Source: CAD feature listing. Evaluate the final solid. Frame: model axes, mm. A direction names the side the tool comes from. Give positions to 0.01 mm unless a question says otherwise; leave off trailing zeros. Order: outer loops, then holes, each group sorted by start corner. A loop starts at its lowest first (then second) coordinate and runs counter-clockwise, first axis right, second up.
```python
from build123d import *

# Parameters (mm, degrees)
SKETCH1_W                    = 1080
SKETCH1_H                    = 33
BASE_FLANGE1_DEPTH           = 2
EDGE_FLANGE1_STRIP_W         = 12
EDGE_FLANGE1_STRIP_H         = 2
EDGE_FLANGE1_STRIP_CUT_DEPTH = 1080
EDGE_FLANGE1_DEPTH           = 1080
SKETCH9_R                    = 7
CUT_EXTRUDE1_DEPTH           = 10
CUT_EXTRUDE2_DEPTH           = 40
CUT_EXTRUDE2_DEPTH_BACK      = 40


# Sheet-metal steps are written as plain solids
with BuildPart() as part:
    # Sketch1 → Base-Flange1 (new body)
    with BuildSketch(Plane.XY):
        Rectangle(SKETCH1_W, SKETCH1_H)
    extrude(amount=-BASE_FLANGE1_DEPTH)

    # Edge-Flange1 strip (across the edge) → Edge-Flange1 strip cut (cut)
    with BuildSketch(Plane(origin=(-540, -16.5, 0), x_dir=(0, 1, 0), z_dir=(1, 0, 0))):
        with Locations((-2, -1)):
            Rectangle(EDGE_FLANGE1_STRIP_W, EDGE_FLANGE1_STRIP_H)
    extrude(amount=EDGE_FLANGE1_STRIP_CUT_DEPTH, mode=Mode.SUBTRACT)

    # Edge-Flange1 section (across the edge) → Edge-Flange1 (add)
    with BuildSketch(Plane(origin=(-540, -16.5, 0), x_dir=(0, 1, 0), z_dir=(1, 0, 0))):
        with BuildLine():
            Line((0, 2), (0, 8))
            Line((0, 8), (2, 8))
            Line((2, 8), (2, 2))
            ThreePointArc((2, 2), (2.585786438, 0.585786438), (4, 0))
            Line((4, 0), (4, -2))
            ThreePointArc((4, -2), (1.171572875, -0.828427125), (0, 2))
        make_face()
    extrude(amount=EDGE_FLANGE1_DEPTH)

    # Sketch9 → Cut-Extrude1 (cut)
    with BuildSketch(Plane.XY):
        with Locations((-930, 2)):
            Circle(SKETCH9_R)
        with Locations((-626, 2)):
            Circle(SKETCH9_R)
        with Locations((-322, 2)):
            Circle(SKETCH9_R)
        with Locations((-18, 2)):
            Circle(SKETCH9_R)
        with Locations((286, 2)):
            Circle(SKETCH9_R)
        with Locations((590, 2)):
            Circle(SKETCH9_R)
        with Locations((894, 2)):
            Circle(SKETCH9_R)
    extrude(amount=-CUT_EXTRUDE1_DEPTH, mode=Mode.SUBTRACT)

    # Sketch10 → Cut-Extrude2 (cut, two sides: drawn at the far end of the back side and taken through both)
    with BuildSketch(Plane.XY.offset(-CUT_EXTRUDE2_DEPTH_BACK)):
        Polygon((-302.377446669, -47.622553331), (-401.622553331, 51.622553331), (-590.417878705, 51.622553331), (-583.65364731, -79.056750642), (-558.625991149, -79.056750642), align=None)
        Polygon((558.625991149, -79.056750642), (302.377446669, -47.622553331), (401.622553331, 51.622553331), (590.417878705, 51.622553331), (583.65364731, -79.056750642), align=None)
    extrude(amount=CUT_EXTRUDE2_DEPTH + CUT_EXTRUDE2_DEPTH_BACK, mode=Mode.SUBTRACT)


solid = part.part
```
1) Reachability of faces 1 (the flat face through (-5, 2, 0)), 2 (the flat face through (-5, 2, -2)) from +Z, -Z, +X, -X, +Y, -Y: full face, straight path, thin tool, end or side. Return the list, or none.
Report:
face 1: +Z, +X, -X, +Y
face 2: -Z, +X, -X, +Y, -Y
2) Section query A-A, the plane x = 286. Return the cut outline in (y, z).
Report:
outline: (-16.5, 2) arc R4 ccw to (-12.5, -2) - (-5, -2) - (-5, 0) - (-12.5, 0) arc R2 cw to (-14.5, 2) - (-14.5, 8) - (-16.5, 8) - close; (9, -2) - (16.5, -2) - (16.5, 0) - (9, 0) - close
3) Section query B-B, the plane z = 3.75. Return the cut outline in (x, y).
Report:
outline: (-335.5, -14.5) - (-333.5, -16.5) - (333.5, -16.5) - (335.5, -14.5) - close
4) Pin query (flat end, axial travel): pin 1 (4 mm diameter, centred on x = -136.5, z = 0, fed in from -Y); pin 2 (3 mm diameter, centred on y = 8, z = 2, fed in from -X); pin 3 (3 mm diameter, centred on y = -6.5, z = -0.5, fed in from -X); pin 4 (1 mm diameter, centred on y = 10, z = -1, fed in from -X). Return the tip coordinate at first contact, or that it passes through.
Report:
pin 1: stops at y = -16.5
pin 2: passes through
pin 3: stops at x = -345
pin 4: stops at x = -360.5
5) Material intervals for L1, parallel to X at y = 4, z = -1.5; L2, parallel to Z at x = 5, y = 1.5; L3, parallel to Y at x = -18, z = -0.55, sorted ascending.
Report:
L1: x = -354 to -328.71, -315.29 to -24.71, -11.29 to 279.29, 292.71 to 354
L2: z = -2 to 0
L3: y = -15.58 to -5, 9 to 16.5
